The model under review builds one solid part; all positions refer to its coordinate system, in mm. Coordinates: 2 decimals unless noted, no trailing zeros. Order: outer loops, then holes, each group sorted by start corner. A loop starts at its lowest first (then second) coordinate and runs counter-clockwise, first axis right, second up. Notation, with made-up numbers: (61, 49.25) -> (81, 49.25) arc R18 ccw to (81, 59.25) -> close; hole circle Ø7 at (53.5, 89). An arc over 180 degrees is marked (long way). Answer as CSV lines item,"result". Start each with the question number.
Autodesk Inventor part; units mm, degrees
ref_plane "YZ Plane" through (0, 0, 0) normal (1, 0, 0) x (0, 1, 0)
ref_plane "XZ Plane" through (0, 0, 0) normal (0, 1, 0) x (-1, 0, 0)
ref_plane "XY Plane" through (0, 0, 0) normal (0, 0, 1) x (1, 0, 0)
sketch "Sketch1" plane through (0, 0, 0) normal (0, 0, 1) x (1, 0, 0)
  line L0 (-37.25, 37.25) -> (37.25, 37.25)
  line L1 (37.25, 37.25) -> (37.25, -37.25)
  line L2 (37.25, -37.25) -> (-37.25, -37.25)
  line L3 (-37.25, -37.25) -> (-37.25, 37.25)
  circle A0 centre (-23.5, 23.5) radius 2
  circle A1 centre (-23.5, -23.5) radius 2
  circle A2 centre (23.5, -23.5) radius 2
  circle A3 centre (23.5, 23.5) radius 2
  circle A4 centre (0, 0) radius 19.1
  circle A5 centre (-32.25, 32.25) radius 2.5
  circle A6 centre (32.25, 32.25) radius 2.5
  circle A7 centre (-32.25, -32.25) radius 2.5
  circle A8 centre (32.25, -32.25) radius 2.5
  dimension "d0" = 4
  dimension "d1" = 4
  dimension "d2" = 4
  dimension "d3" = 4
  dimension "d4" = 38.2
  dimension "d5" = 47
  dimension "d6" = 47
  dimension "d7" = 47
  dimension "d8" = 47
  dimension "d9" = 23.5
  dimension "d10" = 23.5
  dimension "d11" = 23.5
  dimension "d12" = 23.5
  dimension "d13" = 74.5
  dimension "d14" = 74.5
  dimension "d15" = 37.25
  dimension "d16" = 37.25
  dimension "d17" = 5
  dimension "d18" = 5
  dimension "d19" = 5
  dimension "d20" = 5
  dimension "d21" = 64.5
  dimension "d22" = 64.5
  dimension "d23" = 64.5
  dimension "d24" = 64.5
  dimension "d25" = 5
  dimension "d26" = 5
  dimension "d27" = 5
  dimension "d28" = 5
extrude "Extrusion1" add sketch "Sketch1" along normal blind 5
fillet "Fillet1" radius 5 4 edges at (37.25, 37.25, 2.5) (37.25, -37.25, 2.5) (-37.25, 37.25, 2.5) (-37.25, -37.25, 2.5)
properties part number "TurntableMotorBracket"
1) Consider section B-B (y = 0). Give the boundary of the cut face in (x, z).
2) Consider section A-A (x = -23.5). Give the boundary of the cut face in (y, z).
3) Consider section D-D (z = 2.9). Count the separate pieces of the cut face and the enclosed holes in it, plus the area to 3 significant figures.
4) Insertion check: pin 1 Ø3 at (x, y) = (23.5, 23.5) entering from -Z. The pin has a flat end and moves straight along its axis. Give the tip position at first contact, or say it passes through.
5) Wall thickness on L1, parallel to Y at x = 23.5, z = 2.2; L2, parallel to Y at x = 32.25, z = 3.55; L3, parallel to X at y = -31, z = 4.1: over which ranges is each line inside the solid? List them lowest first. Write a range as [from, to].
6) Mouldability with a two-part tool opening along X and no side actions: class faces 1 (the face through (-35.75, 35.82, 2.54)), 2 (the face through (-25.1, -22.3, 2.5)), 3 (the face through (30.41, -33.94, 2.46)), 4 (the face through (0, 37.25, 2)) as released by +X, released by -X, zero draft, split by the parting line, or undercut.
Result:
1,outline,"(-37.25, 0) -> (-19.1, 0) -> (-19.1, 5) -> (-37.25, 5) -> close; (19.1, 0) -> (37.25, 0) -> (37.25, 5) -> (19.1, 5) -> close"
2,outline,"(-37.25, 0) -> (-25.5, 0) -> (-25.5, 5) -> (-37.25, 5) -> close; (-21.5, 0) -> (21.5, 0) -> (21.5, 5) -> (-21.5, 5) -> close; (25.5, 0) -> (37.25, 0) -> (37.25, 5) -> (25.5, 5) -> close"
3,separate pieces,"1"
3,enclosed holes,"9"
3,area,"4,250 mm2"
4,pin 1,"through"
5,L1,"[-37.25, -25.5], [-21.5, 21.5], [25.5, 37.25]"
5,L2,"[-37.25, -34.75], [-29.75, 29.75], [34.75, 37.25]"
5,L3,"[-37.25, -34.42], [-30.08, 30.08], [34.42, 37.25]"
6,face 1,"released by -X"
6,face 2,"undercut"
6,face 3,"undercut"
6,face 4,"zero draft"
